Can you work these out from the model? Positions are in its coordinate system, mm. A direction names the side the tool comes from. Give positions to 0.01 mm unless a question says otherwise; leave off trailing zeros. Write each loop counter-clockwise with the first axis right and the second up, starting at its lowest first coordinate (ties: lowest second). Pieces come first, ordered by that corner, then holes.
```python
from build123d import *

# Parameters (mm, degrees)
SKETCH_R        = 22.5
PAD_DEPTH       = 3
SKETCH001_R     = 22.5
SKETCH001_R_2   = 20.3
PAD001_DEPTH    = 5
SKETCH002_R     = 10
SKETCH002_R_2   = 3.6
PAD002_DEPTH    = 4
SKETCH003_R     = 3
POCKET_DEPTH    = 8.001
FILLET_R        = 2
CHAMFER_SIZE    = 1
CHAMFER001_SIZE = 1


with BuildPart() as part:
    # Sketch → Pad (new body)
    with BuildSketch(Plane.XY):
        Circle(SKETCH_R)
    extrude(amount=PAD_DEPTH)

    # Sketch001 (on Face3 of Pad) → Pad001 (join)
    with BuildSketch(Plane.XY.offset(3)):
        Circle(SKETCH001_R)
        Circle(SKETCH001_R_2, mode=Mode.SUBTRACT)
    extrude(amount=PAD001_DEPTH)

    # Sketch002 (on Face5 of Pad001) → Pad002 (join)
    with BuildSketch(Plane.XY.offset(3)):
        Circle(SKETCH002_R)
        Circle(SKETCH002_R_2, mode=Mode.SUBTRACT)
    extrude(amount=PAD002_DEPTH)

    # Sketch003 (on Face1 of Pad002) → Pocket (cut, through all)
    with BuildSketch(Plane(origin=(0, 0, 0), x_dir=(1, 0, 0), z_dir=(0, 0, -1))):
        with Locations((-6.5, 6.5)):
            Circle(SKETCH003_R)
        with Locations((-6.5, -6.5)):
            Circle(SKETCH003_R)
        with Locations((6.5, -6.5)):
            Circle(SKETCH003_R)
        with Locations((6.5, 6.5)):
            Circle(SKETCH003_R)
    extrude(amount=-POCKET_DEPTH, mode=Mode.SUBTRACT)

    # Fillet
    fillet_edges = [part.edges().sort_by_distance(p)[0] for p in [
        (-22.5, 0, 0),
    ]]
    fillet(fillet_edges, radius=FILLET_R)

    # Chamfer
    chamfer_edges = [part.edges().sort_by_distance(p)[0] for p in [
        (-20.3, 0, 8),
    ]]
    chamfer(chamfer_edges, length=CHAMFER_SIZE)

    # Chamfer001
    chamfer001_edges = [part.edges().sort_by_distance(p)[0] for p in [
        (-3.6, 0, 7),
    ]]
    chamfer(chamfer001_edges, length=CHAMFER001_SIZE)


solid = part.part
```
1) Suppose I cut it at A-A on z = 5. Write out the boundary of the cut face in (x, y), plus the area to 3 significant figures.
Values follow:
outline: circle Ø45 at (0, 0); (-8.86, -4.64) arc R3 cw (long way) to (-4.64, -8.86) arc R10 ccw to (4.64, -8.86) arc R3 cw (long way) to (8.86, -4.64) arc R10 ccw to (8.86, 4.64) arc R3 cw (long way) to (4.64, 8.86) arc R10 ccw to (-4.64, 8.86) arc R3 cw (long way) to (-8.86, 4.64) arc R10 ccw to start; hole circle Ø40.6 at (0, 0); hole circle Ø7.2 at (0, 0)
area: 497 mm2
2) Please list where these lines run through material, in increasing order: L1, parallel to Y at x = 0, z = 3.85; L2, parallel to X at y = 1, z = 6.75; L3, parallel to Y at x = -6.5, z = 2.
Values follow:
L1: y = -22.5 to -20.3, -10 to -3.6, 3.6 to 10, 20.3 to 22.5
L2: x = -22.48 to -20.28, -9.95 to -4.23, 4.23 to 9.95, 20.28 to 22.48
L3: y = -21.54 to -9.5, -3.5 to 3.5, 9.5 to 21.54
3) For pin 1 Ø2 at (x, z) = (17.5, 1) entering from -Y; pin 2 Ø10 at (x, y) = (-2.5, -2.5) entering from +Z; pin 3 Ø3 at (x, y) = (6.5, 12.5) entering from +Z, each with a flat end and sliding along its axis, tell me the tip position at first contact or that it passes through.
Values follow:
pin 1: stops at y = -15.07
pin 2: stops at z = 7
pin 3: stops at z = 3
4) For faces 4 (the face through (-16.11, -12.35, 4.97)), 5 (the face through (8, -20, 8)), which set-ups out of +Z, -Z, +X, -X, +Y, -Y let a thin tool reach every point of the face, with its end or its side?
Values follow:
face 4: +Z
face 5: +Z, +X, -X, +Y, -Y
5) If we mould it in two halves opening along X, with no side actions, what happens to faces 1 (the face through (-9.3, -4.2, 3)), 2 (the face through (10.382, -19.961, 4.958)), 3 (the face through (0, 0, 0))? For each: +X half, -X half, draft (parallel to the pull), parting line (faces both ways), or undercut.
Values follow:
face 1: undercut
face 2: parting line
face 3: draft
6) Suppose I cut it at B-B on x = 0. Write out the boundary of the cut face in (y, z), plus the area to 3 significant figures.
Values follow:
outline: (-22.5, 2) arc R2 ccw to (-20.5, 0) - (20.5, 0) arc R2 ccw to (22.5, 2) - (22.5, 8) - (21.3, 8) - (20.3, 7) - (20.3, 3) - (10, 3) - (10, 7) - (4.6, 7) - (3.6, 6) - (3.6, 3) - (-3.6, 3) - (-3.6, 6) - (-4.6, 7) - (-10, 7) - (-10, 3) - (-20.3, 3) - (-20.3, 7) - (-21.3, 8) - (-22.5, 8) - close
area: 204 mm2
7) Suppose I cut it at D-D on y = -6.5. State how many separate pieces and enclosed holes the cut face has, plus the area to 3 significant figures.
Values follow:
separate pieces: 3
enclosed holes: 0
area: 141 mm2
